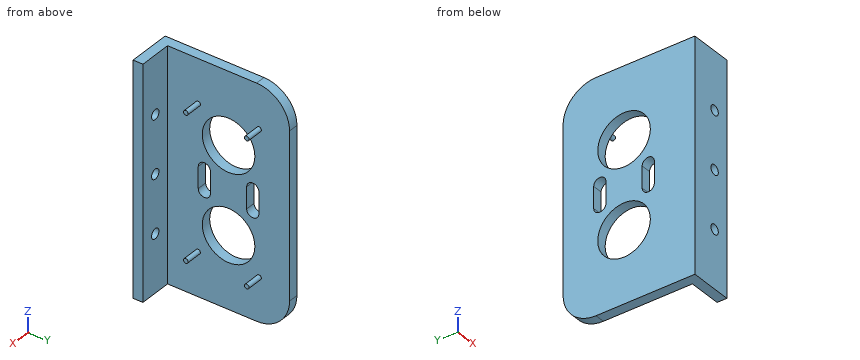
from build123d import *

# Parameters (mm, degrees)
BOSS_EXTRUDE1_DEPTH = 70
SKETCH2_R           = 7.975
CUT_EXTRUDE9_DEPTH  = 82.240384046
SKETCH2_12_R        = 7.975
CUT_EXTRUDE10_DEPTH = 82.240384046
FILLET1_R           = 10
FILLET2_R           = 10
SKETCH3_R           = 1.5
CUT_EXTRUDE11_DEPTH = 81.237148504
CUT_EXTRUDE12_DEPTH = 82.663945533
SKETCH6_R           = 0.7
BOSS_EXTRUDE2_DEPTH = 8


# Read off the part's stored shape, not the designer's step: Boss-Extrude1
with BuildPart() as part:
    # Boss-Extrude1 outline → Boss-Extrude1 (new body)
    with BuildSketch(Plane.XY):
        Polygon((-10, 40), (-13, 40), (-13, 0), (0, 0), (0, 3), (-10, 3), align=None)
    extrude(amount=BOSS_EXTRUDE1_DEPTH)

    # Sketch2 → Cut-Extrude9 (cut, through all)
    with BuildSketch(Plane(origin=(-10, 0, 0), x_dir=(0, 0, -1), z_dir=(1, 0, 0))):
        with Locations((-48.25, 21.5)):
            Circle(SKETCH2_R)
    extrude(amount=-CUT_EXTRUDE9_DEPTH, mode=Mode.SUBTRACT)

    # Sketch2<12> → Cut-Extrude10 (cut, through all)
    with BuildSketch(Plane(origin=(-10, 0, 0), x_dir=(0, 0, -1), z_dir=(1, 0, 0))):
        with Locations((-21.75, 21.5)):
            Circle(SKETCH2_12_R)
    extrude(amount=-CUT_EXTRUDE10_DEPTH, mode=Mode.SUBTRACT)

    # Fillet1
    fillet1_edges = [part.edges().sort_by_distance(p)[0] for p in [
        (-11.5, 40, 70),
    ]]
    fillet(fillet1_edges, radius=FILLET1_R)

    # Fillet2
    fillet2_edges = [part.edges().sort_by_distance(p)[0] for p in [
        (-11.5, 40, 0),
    ]]
    fillet(fillet2_edges, radius=FILLET2_R)

    # Sketch3 → Cut-Extrude11 (cut, through all)
    with BuildSketch(Plane(origin=(0, 3, 0), x_dir=(1, 0, 0), z_dir=(0, 1, 0))):
        with Locations(Location((-5, -35, 0), (0, 0, 270))):
            Circle(SKETCH3_R)
        with Locations(Location((-5, -52.5, 0), (0, 0, 270))):
            Circle(SKETCH3_R)
        with Locations(Location((-5, -17.5, 0), (0, 0, 270))):
            Circle(SKETCH3_R)
    extrude(amount=-CUT_EXTRUDE11_DEPTH, mode=Mode.SUBTRACT)

    # Sketch4 → Cut-Extrude12 (cut, through all)
    with BuildSketch(Plane.ZY.offset(13)):
        with BuildLine():
            Line((38.3, 27), (31.8, 27))
            ThreePointArc((31.8, 27), (29.95, 28.85), (31.8, 30.7))
            Line((31.8, 30.7), (38.3, 30.7))
            ThreePointArc((38.3, 30.7), (40.15, 28.85), (38.3, 27))
        make_face()
        with BuildLine():
            Line((38.3, 16), (31.8, 16))
            ThreePointArc((31.8, 16), (29.95, 14.15), (31.8, 12.3))
            Line((31.8, 12.3), (38.3, 12.3))
            ThreePointArc((38.3, 12.3), (40.15, 14.15), (38.3, 16))
        make_face()
    extrude(amount=-CUT_EXTRUDE12_DEPTH, mode=Mode.SUBTRACT)

    # Sketch6 → Boss-Extrude2 (add)
    with BuildSketch(Plane.ZY.offset(13)):
        with Locations(Location((56.75, 30.75, 0), (0, 0, 270))):
            Circle(SKETCH6_R)
        with Locations(Location((56.75, 12.25, 0), (0, 0, 270))):
            Circle(SKETCH6_R)
        with Locations(Location((13.25, 30.75, 0), (0, 0, 270))):
            Circle(SKETCH6_R)
        with Locations(Location((13.25, 12.25, 0), (0, 0, 270))):
            Circle(SKETCH6_R)
    extrude(amount=-BOSS_EXTRUDE2_DEPTH)


solid = part.part
Input: part model. Units: mm. Frame: model coordinates. Coordinates: 2 decimals unless noted, no trailing zeros. Loops run counter-clockwise (first coordinate to the right, second up) from the corner with the lowest first, then second, coordinate; pieces in that order, holes last. Notation, with made-up numbers: (-31, -7.5) -> (-23, -7.5) arc R28 cw to (-23, 29.5) -> close; hole circle Ø10 at (44.25, 36.25). An arc over 180 degrees is marked (long way). Write each question's results on one line, items separated by ' | '. Start each with the question number.
Q1. Section C-C, the plane z = 21.75. Return the cut outline in (x, y) (3 decimals), plus the area to 3 significant figures.
Q2. Section A-A, the plane z = 35. Return the cut outline in (x, y), plus the area to 3 significant figures.
Q3. Section D-D, the plane z = 52.5. Return the cut outline in (x, y).
Q4. Pin query (flat end, axial travel): pin 1 (1.5 mm diameter, centred on y = 12, z = 13, fed in from +X); pin 2 (3 mm diameter, centred on y = 30.5, z = 36.5, fed in from -X); pin 3 (6 mm diameter, centred on x = -5.5, y = 11, fed in from +Z); pin 4 (3.5 mm diameter, centred on x = -5, z = 52.5, fed in from +Y). Return the tip coordinate at first contact, or that it passes through.
Q5. Section B-B, the plane y = 20. Return the cut outline in (x, z).
Q6. Ray query, line 1 (Y direction, x = -12, z = 36.5); line 2 (X direction, y = 2.1, z = 35); line 3 (Y direction, x = -11, z = 21.75) (3 decimals). Return the intervals inside material, ascending. Write a range as from..to.
Found:
1) outline: (-13, 0) -> (0, 0) -> (0, 3) -> (-10, 3) -> (-10, 13.525) -> (-13, 13.525) -> close; (-13, 29.475) -> (-10, 29.475) -> (-10, 40) -> (-13, 40) -> close | area: 102 mm2
2) outline: (-13, 0) -> (-6.5, 0) -> (-6.5, 3) -> (-10, 3) -> (-10, 12.3) -> (-13, 12.3) -> close; (-13, 16) -> (-10, 16) -> (-10, 27) -> (-13, 27) -> close; (-13, 30.7) -> (-10, 30.7) -> (-10, 40) -> (-13, 40) -> close; (-3.5, 0) -> (0, 0) -> (0, 3) -> (-3.5, 3) -> close | area: 119 mm2
3) outline: (-13, 0) -> (-6.5, 0) -> (-6.5, 3) -> (-10, 3) -> (-10, 14.75) -> (-13, 14.75) -> close; (-13, 28.25) -> (-10, 28.25) -> (-10, 40) -> (-13, 40) -> close; (-3.5, 0) -> (0, 0) -> (0, 3) -> (-3.5, 3) -> close
4) pin 1: x = -5 | pin 2: x = -13 | pin 3: z = 57.45 | pin 4: y = 3
5) outline: (-13, 0) -> (-10, 0) -> (-10, 13.92) -> (-13, 13.92) -> close; (-13, 29.58) -> (-10, 29.58) -> (-10, 40.42) -> (-13, 40.42) -> close; (-13, 56.08) -> (-10, 56.08) -> (-10, 70) -> (-13, 70) -> close
6) line 1: 0..12.3, 16..27, 30.7..40 | line 2: -13..-6.5, -3.5..0 | line 3: 0..13.525, 29.475..40
